from build123d import *

# Parameters (mm, degrees)
BOSS_EXTRUDE1_DEPTH     = 9.525
SKETCH12_R              = 2.75
CUT_EXTRUDE2_DEPTH      = 230.653490339
CUT_EXTRUDE3_DEPTH      = 285.764333485
CUT_EXTRUDE3_DEPTH_BACK = 285.764333485
SKETCH13_R              = 2.75


with BuildPart() as part:
    # Sketch1 → Boss-Extrude1 (new, symmetric)
    with BuildSketch(Plane.XY):
        with BuildLine():
            Line((45, 45), (45, 240))
            ThreePointArc((45, 240), (36.213203436, 261.213203436), (15, 270))
            Line((15, 270), (-15, 270))
            ThreePointArc((-15, 270), (-36.213203436, 261.213203436), (-45, 240))
            Line((-45, 240), (-45, 45))
            Line((-45, 45), (-41.825, 45))
            Line((-41.825, 45), (-41.825, 240))
            ThreePointArc((-41.825, 240), (-33.968139405, 258.968139405), (-15, 266.825))
            Line((-15, 266.825), (15, 266.825))
            ThreePointArc((15, 266.825), (33.968139405, 258.968139405), (41.825, 240))
            Line((41.825, 240), (41.825, 45))
            Line((41.825, 45), (45, 45))
        make_face()
    extrude(amount=BOSS_EXTRUDE1_DEPTH, both=True)

    # Sketch12 → Cut-Extrude2 (cut, through all)
    with BuildSketch(Plane(origin=(0, 270, 0), x_dir=(1, 0, 0), z_dir=(0, 1, 0))):
        with Locations(Location((0, 0, 0), (0, 0, 270))):
            Circle(SKETCH12_R)
        with Locations(Location((-10, 0, 0), (0, 0, 270))):
            Circle(SKETCH12_R)
        with Locations(Location((10, 0, 0), (0, 0, 270))):
            Circle(SKETCH12_R)
    extrude(amount=-CUT_EXTRUDE2_DEPTH, mode=Mode.SUBTRACT)

    # Sketch13 → Cut-Extrude3 (cut, two sides: drawn at the far end of the back side and taken through both)
    with BuildSketch(Plane(origin=(45, 0, 0), x_dir=(0, 0, -1), z_dir=(1, 0, 0)).offset(-CUT_EXTRUDE3_DEPTH_BACK)):
        with Locations(Location((0, 125, 0), (0, 0, 90))):
            Circle(SKETCH13_R)
        with Locations(Location((0, 55, 0), (0, 0, 90))):
            Circle(SKETCH13_R)
    extrude(amount=CUT_EXTRUDE3_DEPTH + CUT_EXTRUDE3_DEPTH_BACK, mode=Mode.SUBTRACT)


solid = part.part
Could you check a few things on this model? Use its own coordinates, in mm. A direction names the side the tool comes from. Round coordinates to 2 decimals unless told otherwise and drop trailing zeros. Order: outer loops, then holes, each group sorted by start corner. A loop starts at its lowest first (then second) coordinate and runs counter-clockwise, first axis right, second up.
Q1. Please list where these lines run through material, in increasing order: probe 1 along X at (y, z) = (181, 3) (3 decimals); probe 2 along Z at (x, y) = (43, 125) (3 decimals); probe 3 along X at (y, z) = (254.5, 6.25).
Geometry says:
probe 1: x = -45 to -41.825, 41.825 to 45
probe 2: z = -9.525 to -2.75, 2.75 to 9.525
probe 3: x = -41.26 to -37.57, 37.57 to 41.26
Q2. Imagine slicing it at C-C, the plane x = 10. List the corners of the cut face in (y, z) for me (3 decimals).
Geometry says:
outline: (266.825, -9.525) - (270, -9.525) - (270, -2.75) - (266.825, -2.75) - close; (266.825, 2.75) - (270, 2.75) - (270, 9.525) - (266.825, 9.525) - close
Q3. Imagine slicing it at B-B, the plane y = 125. List the corners of the cut face in (x, z) for me (3 decimals), then the cut area to 3 significant figures.
Geometry says:
outline: (-45, -9.525) - (-41.825, -9.525) - (-41.825, -2.75) - (-45, -2.75) - close; (-45, 2.75) - (-41.825, 2.75) - (-41.825, 9.525) - (-45, 9.525) - close; (41.825, -9.525) - (45, -9.525) - (45, -2.75) - (41.825, -2.75) - close; (41.825, 2.75) - (45, 2.75) - (45, 9.525) - (41.825, 9.525) - close
area: 86.0 mm2
Q4. Thinking about a two-plate mould opening in Y: for faces 1 (the face through (-43.43, 127.62, 0.83)), 2 (the face through (-2.685, 268.435, -0.596)), 3 (the face through (4, 270, 0)), which applies, released by +Y, released by -Y, zero draft, split by the parting line, or undercut?
Geometry says:
face 1: undercut
face 2: zero draft
face 3: released by +Y
Q5. Imagine slicing it at A-A, the plane y = 201. List the corners of the cut face in (x, z) for me (3 decimals), then the cut area to 3 significant figures.
Geometry says:
outline: (-45, -9.525) - (-41.825, -9.525) - (-41.825, 9.525) - (-45, 9.525) - close; (41.825, -9.525) - (45, -9.525) - (45, 9.525) - (41.825, 9.525) - close
area: 121 mm2
Q6. Which directions (+Z, -Z, +X, -X, +Y, -Y) give clear straight access to the entire face, cutting with the end or side of a thin tool? Please do faces 4 (the face through (-41.825, 141, 0)), 5 (the face through (12.727, 268.435, -0.358)).
Geometry says:
face 4: +Z, -Z, -Y
face 5: +Y, -Y
Q7. I'm going to push flat-ended pins straight in: P1, Ø6.5, axis at x = -10, z = 0, coming from the -Y side (3 decimals); P2, Ø5, axis at y = 125, z = 0, coming from the +X side (3 decimals); P3, Ø3, axis at x = -20, z = 0.5, coming from the +Y side. Where does each tip first touch, or does it pass through?
Geometry says:
P1: stops at y = 266.825
P2: passes through
P3: stops at y = 269.8
Q8. Imagine slicing it at D-D, the plane z = 0. State how many separate pieces and enclosed holes the cut face has, then the cut area to 3 significant figures.
Geometry says:
separate pieces: 8
enclosed holes: 0
area: 1,490 mm2
